The listing builds one solid part. Answer for the finished solid, in the listing's coordinates (mm). A direction names the side the tool comes from. Give positions to 0.01 mm unless a question says otherwise; leave off trailing zeros. Order: outer loops, then holes, each group sorted by start corner. A loop starts at its lowest first (then second) coordinate and runs counter-clockwise, first axis right, second up. Notation, with made-up numbers: (1, 72.5) - (36, 72.5) arc R14 ccw to (36, 88.5) - close; hole circle Ø1 at (10.5, 74.25). An arc over 180 degrees is marked (long way). Answer in a Markdown table with one row per item. Add a question column.
Autodesk Inventor part; units mm, degrees
ref_plane "YZ Plane" through (0, 0, 0) normal (1, 0, 0) x (0, 1, 0)
ref_plane "XZ Plane" through (0, 0, 0) normal (0, 1, 0) x (-1, 0, 0)
ref_plane "XY Plane" through (0, 0, 0) normal (0, 0, 1) x (1, 0, 0)
sketch "Sketch1" plane through (0, 0, 0) normal (0, 0, 1) x (1, 0, 0)
  line L0 (64.6, 10) -> (64.6, 9.5)
  line L1 (64.6, 9.5) -> (65.7, 9.5)
  line L2 (65.7, 9.5) -> (65.7, 10)
  line L3 (65.7, 10) -> (80.7, 10)
  line L4 (80.7, 10) -> (80.7, 9.5)
  line L5 (80.7, 9.5) -> (81.8, 9.5)
  line L6 (81.8, 9.5) -> (81.8, 10)
  line L7 (81.8, 10) -> (84.8, 10)
  line L8 (84.8, 10) -> (84.8, 0)
  line L9 (84.8, 0) -> (0, 0)
  line L10 (0, 10) -> (0, 0)
  line L11 (64.6, 10) -> (49.6, 10)
  line L12 (49.6, 10) -> (49.6, 9.5)
  line L13 (49.6, 9.5) -> (48.5, 9.5)
  line L14 (48.5, 9.5) -> (48.5, 10)
  line L15 (0, 10) -> (2, 10)
  line L16 (2, 10) -> (2, 9.5)
  line L17 (2, 9.5) -> (3.1, 9.5)
  line L18 (3.1, 9.5) -> (3.1, 10)
  line L19 (3.1, 10) -> (48.5, 10)
  dimension "d3" = 1.1
  dimension "d5" = 1.1
  dimension "d6" = 10
  dimension "d12" = 3
  dimension "d20" = 0.5
  dimension "d21" = 0.5
  dimension "d22" = 0.5
  dimension "d23" = 15
  dimension "d32" = 64.6
  dimension "d33" = 15
  dimension "d34" = 1.1
  dimension "d35" = 0.5
  dimension "d36" = 1.1
  dimension "d37" = 0.5
  dimension "d38" = 2
revolve "Revolution1" add sketch "Sketch1" angle 360 about axis through (84.8, 0, 0) along (-1, 0, 0)
properties part number "Center Axle" material "Steel, Mild"
(1) The mould has two halves that part along X. Classify faces 3 (the face through (84.8, 0, 0)), 4 (the face through (83.32, -2.17, -9.76)), 5 (the face through (65.7, 9, 4)), 6 (the face through (3.1, 9, 4)): +X half, -X half, draft (parallel to the pull), parting line (faces both ways), or undercut.
(2) For faces 1 (the face through (57, -2.17, 9.76)), 2 (the face through (81.8, 9, 4)), determine the directions among +Z, -Z, +X, -X, +Y, -Y from which every point of the face is accessible in a straight line to the end or side of a thin tool.
(3) Find section A-A, the plane x = 40. Write down the section's boundary in (y, z).
(4) Straight lines are drawn through the part: line 1 (X direction, y = -5.75, z = 7.75); line 2 (Z direction, x = 33.5, y = 0); line 3 (Y direction, x = 14, z = 0.5). For each, find the intervals that lie inside material, in ascending order.
(5) Each of these flat-tipped pins is pushed along its axis until it touches: P1, Ø5, axis at x = 62, y = 3.5, coming from the -Z side; P2, Ø12, axis at y = 5.5, z = 6.5, coming from the -X side; P3, Ø3, axis at x = 74, z = -7, coming from the +Y side; P4, Ø1, axis at x = 41, y = -2.5, coming from the -Z side. Where does it stop, or does it pass through?
Answer key:
| question | item | result |
|---|---|---|
| 1 | face 3 | +X half |
| 1 | face 4 | draft |
| 1 | face 5 | undercut |
| 1 | face 6 | undercut |
| 2 | face 1 | +X, -X |
| 2 | face 2 | none |
| 3 | outline | circle Ø20 at (0, 0) |
| 4 | line 1 | 0 to 2, 3.1 to 48.5, 49.6 to 64.6, 65.7 to 80.7, 81.8 to 84.8 |
| 4 | line 2 | -10 to 10 |
| 4 | line 3 | -9.99 to 9.99 |
| 5 | P1 | z = -9.95 |
| 5 | P2 | x = 0 |
| 5 | P3 | y = 8.35 |
| 5 | P4 | z = -9.8 |
